Autodesk Inventor part; units mm, degrees
ref_plane "작업 평면1" through (0, 1.7, 0) normal (0, 1, 0) x (1, 0, 0)
ref_plane "YZ Plane" through (0, 0, 0) normal (1, 0, 0) x (0, 1, 0)
ref_plane "XZ Plane" through (0, 0, 0) normal (0, 1, 0) x (-1, 0, 0)
sketch "스케치1" plane through (0, 0, 0) normal (0, 1, 0) x (-1, 0, 0)
  line L0 (-32.5919, 13.5) -> (-13.5, 32.5919)
  line L1 (-13.5, 32.5919) -> (13.5, 32.5919)
  line L2 (13.5, 32.5919) -> (32.5919, 13.5)
  line L3 (32.5919, 13.5) -> (32.5919, -13.5)
  line L4 (32.5919, -13.5) -> (13.5, -32.5919)
  line L5 (13.5, -32.5919) -> (-13.5, -32.5919)
  line L6 (-13.5, -32.5919) -> (-32.5919, -13.5)
  line L7 (-32.5919, -13.5) -> (-32.5919, 13.5)
  line L8 (34.9919, 14.4941) -> (34.9919, -14.4941)
  line L9 (34.9919, -14.4941) -> (14.4941, -34.9919)
  line L10 (14.4941, -34.9919) -> (-14.4941, -34.9919)
  line L11 (-14.4941, -34.9919) -> (-34.9919, -14.4941)
  line L12 (-34.9919, -14.4941) -> (-34.9919, 14.4941)
  line L13 (-34.9919, 14.4941) -> (-14.4941, 34.9919)
  line L14 (-14.4941, 34.9919) -> (14.4941, 34.9919)
  line L15 (14.4941, 34.9919) -> (34.9919, 14.4941)
  point P0 (0, 0)
  point P1 (0, 0)
  point P2 (0, 0)
  dimension "d0" = 27
  dimension "d1" = 2.4
extrude "돌출1" add sketch "스케치1" along normal blind 3.4 contours L0 L1 L2 L3 L4 L5 L6 L7 | L8 L9 L10 L11 L12 L13 L14 L15
sketch "스케치3" plane through (0, 0, 0) normal (0, -1, 0) x (1, 0, 0)
  line L0 (-13.5, 32.5919) -> (13.5, 32.5919)
  line L1 (13.5, 32.5919) -> (32.5919, 13.5)
  line L2 (32.5919, 13.5) -> (32.5919, -13.5)
  line L3 (32.5919, -13.5) -> (13.5, -32.5919)
  line L4 (13.5, -32.5919) -> (-13.5, -32.5919)
  line L5 (-13.5, -32.5919) -> (-32.5919, -13.5)
  line L6 (-32.5919, -13.5) -> (-32.5919, 13.5)
  line L7 (-32.5919, 13.5) -> (-13.5, 32.5919)
  line L8 (-13.9971, 33.7919) -> (13.9971, 33.7919)
  line L9 (13.9971, 33.7919) -> (33.7919, 13.9971)
  line L10 (33.7919, 13.9971) -> (33.7919, -13.9971)
  line L11 (33.7919, -13.9971) -> (13.9971, -33.7919)
  line L12 (13.9971, -33.7919) -> (-13.9971, -33.7919)
  line L13 (-13.9971, -33.7919) -> (-33.7919, -13.9971)
  line L14 (-33.7919, -13.9971) -> (-33.7919, 13.9971)
  line L15 (-33.7919, 13.9971) -> (-13.9971, 33.7919)
  line L16 (-13.1686, 31.7919) -> (13.1686, 31.7919)
  line L17 (13.1686, 31.7919) -> (31.7919, 13.1686)
  line L18 (31.7919, 13.1686) -> (31.7919, -13.1686)
  line L19 (31.7919, -13.1686) -> (13.1686, -31.7919)
  line L20 (13.1686, -31.7919) -> (-13.1686, -31.7919)
  line L21 (-13.1686, -31.7919) -> (-31.7919, -13.1686)
  line L22 (-31.7919, -13.1686) -> (-31.7919, 13.1686)
  line L23 (-31.7919, 13.1686) -> (-13.1686, 31.7919)
  point P0 (0, 0)
  point P1 (0, 0)
  point P2 (0, 0)
  point P3 (0, 0)
  dimension "d8" = 27
  dimension "d9" = 1.2
  dimension "d19" = 0.8
extrude "돌출3" cut sketch "스케치3" against normal blind 1.2 contours L0 L1 L2 L3 L4 L5 L6 L7 | L8 L9 L10 L11 L12 L13 L14 L15 | L16 L17 L18 L19 L20 L21 L22 L23
sketch "스케치4" plane through (0, 3.4, 0) normal (0, 1, 0) x (1, 0, 0)
  line L0 (11.926, -28.7919) -> (-11.926, -28.7919)
  line L1 (-11.926, -28.7919) -> (-28.7919, -11.926)
  line L2 (-28.7919, -11.926) -> (-28.7919, 11.926)
  line L3 (-28.7919, 11.926) -> (-11.926, 28.7919)
  line L4 (-11.926, 28.7919) -> (11.926, 28.7919)
  line L5 (11.926, 28.7919) -> (28.7919, 11.926)
  line L6 (28.7919, 11.926) -> (28.7919, -11.926)
  line L7 (28.7919, -11.926) -> (11.926, -28.7919)
  line L8 (-31.7919, -13.1686) -> (-31.7919, 13.1686)
  point P0 (0, 0)
  point P1 (0, 0)
  dimension "d21" = 3
extrude "돌출4" cut sketch "스케치4" against normal blind 5
ref_plane "작업 평면1" through (0, 1.7, 0) normal (0, 1, 0) x (1, 0, 0)
sketch "스케치6" plane through (0, 0, 0) normal (0, -1, 0) x (1, 0, 0)
  line L0 (28.7919, -11.926) -> (11.926, -28.7919)
  line L1 (11.926, -28.7919) -> (-11.926, -28.7919)
  line L2 (-11.926, -28.7919) -> (-28.7919, -11.926)
  line L3 (-28.7919, -11.926) -> (-28.7919, 11.926)
  line L4 (-28.7919, 11.926) -> (-11.926, 28.7919)
  line L5 (-11.926, 28.7919) -> (11.926, 28.7919)
  line L6 (11.926, 28.7919) -> (28.7919, 11.926)
  line L7 (28.7919, 11.926) -> (28.7919, -11.926)
  line L8 (31.7919, 13.1686) -> (13.1686, 31.7919)
  line L9 (13.1686, 31.7919) -> (-13.1686, 31.7919)
  line L10 (-13.1686, 31.7919) -> (-31.7919, 13.1686)
  line L11 (-31.7919, 13.1686) -> (-31.7919, -13.1686)
  line L12 (-31.7919, -13.1686) -> (-13.1686, -31.7919)
  line L13 (-13.1686, -31.7919) -> (13.1686, -31.7919)
  line L14 (13.1686, -31.7919) -> (31.7919, -13.1686)
  line L15 (31.7919, -13.1686) -> (31.7919, 13.1686)
  point P0 (0, 0)
extrude "돌출7" cut sketch "스케치6" against normal blind 1.2
mirror "미러2" about plane through (0, 1.7, 0) normal (0, 1, 0) of "돌출7", "돌출3"
chamfer "모따기22" distance 0.5 distance2 3 2 edges at (-20.3589, 1.2, -20.3589) (-20.3589, 2.2, -20.3589) measured on face at (-17.548, 1.8667, -23.1699)
chamfer "모따기23" distance 0.5 distance2 3 2 edges at (-28.7919, 1.2, 0) (-28.7919, 2.2, 0) measured on face at (-28.7919, 1.6998, 3.9753)
chamfer "모따기24" distance 0.5 distance2 3 2 edges at (-20.3589, 1.2, 20.3589) (-20.3589, 2.2, 20.3589) measured on face at (-17.548, 1.6998, 23.1699)
chamfer "모따기25" distance 0.5 distance2 3 2 edges at (0, 1.2, 28.7919) (0, 2.2, 28.7919) measured on face at (3.9753, 1.6998, 28.7919)
chamfer "모따기26" distance 0.5 distance2 3 2 edges at (20.3589, 1.2, 20.3589) (20.3589, 2.2, 20.3589) measured on face at (23.1699, 1.7002, 17.548)
chamfer "모따기27" distance 0.5 distance2 3 2 edges at (28.7919, 1.2, 0) (28.7919, 2.2, 0) measured on face at (28.7919, 1.7002, -3.9753)
chamfer "모따기28" distance 0.5 distance2 3 2 edges at (20.3589, 1.2, -20.3589) (20.3589, 2.2, -20.3589) measured on face at (17.548, 1.7002, -23.1699)
chamfer "모따기29" distance 0.5 distance2 3 2 edges at (0, 1.2, -28.7919) (0, 2.2, -28.7919) measured on face at (-3.9753, 2.0335, -28.7919)
properties part number "OV-PAM_ring_2"
Design review of the part built by this model. Coordinates are the model's own, in mm. A direction names the side the tool comes from. Give positions to 0.01 mm unless a question says otherwise; leave off trailing zeros. Order: outer loops, then holes, each group sorted by start corner. A loop starts at its lowest first (then second) coordinate and runs counter-clockwise, first axis right, second up.
1. To check wall thickness, follow L1, parallel to Z at x = -12.5, y = 1; L2, parallel to Z at x = -18.5, y = 0.25. State the ranges of each line that lie inside material, in increasing order.
Solution:
L1: z = -34.99 to -33.79, 33.79 to 34.99
L2: z = -30.99 to -29.29, 29.29 to 30.99
2. Add section C-C, the plane x = -30. State the section outline as (y, z) points.
Solution:
outline: (0, -19.49) - (3.4, -19.49) - (3.4, -17.79) - (2.2, -17.79) - (2.2, -14.96) - (1.9, -12.43) - (1.9, 12.43) - (2.2, 14.96) - (2.2, 17.79) - (3.4, 17.79) - (3.4, 19.49) - (0, 19.49) - (0, 17.79) - (1.2, 17.79) - (1.2, 14.96) - (1.5, 12.43) - (1.5, -12.43) - (1.2, -14.96) - (1.2, -17.79) - (0, -17.79) - close
3. For pin 1 Ø5 at (x, z) = (28, 14.5) entering from -Y; pin 2 Ø20.5 at (x, z) = (14.5, 7.5) entering from +Y; pin 3 Ø1.5 at (x, y) = (-19.5, 2) entering from +Z, all flat-tipped, find the tip position at first contact; note any pin that passes through.
Solution:
pin 1: stops at y = 1.2
pin 2: passes through
pin 3: stops at z = 30.74
4. Mouldability with a two-part tool opening along Z and no side actions: class faces 1 (the flat face through (-30.313, 1.446, -0.184)), 2 (the flat face through (-24.6, 1.676, 24.886)), 3 (the flat face through (0, 2, -34.992)), 4 (the flat face through (23.76, 0.59, 24.03)) as +Z half, -Z half, draft (parallel to the pull), parting line (faces both ways), or undercut.
Solution:
face 1: undercut
face 2: +Z half
face 3: -Z half
face 4: undercut
5. Tool access review of faces 5 (the flat face through (21.304, 1.954, 21.565)), 6 (the flat face through (-24.886, 1.676, -24.6)), 7 (the flat face through (-21.305, 1.446, -21.563)): name each direction out of +Z, -Z, +X, -X, +Y, -Y from which nothing blocks a thin tool from reaching the whole face with its end or side.
Solution:
face 5: +Y
face 6: -Z, -X, +Y, -Y
face 7: -Y
